Verification items for this drawing (mm, ordinates from the low corner). Coordinates: 2 decimals unless noted, no trailing zeros. Write each loop counter-clockwise with the first axis right and the second up, starting at its lowest first coordinate (ties: lowest second). Pieces come first, ordered by that corner, then holes. Notation, with made-up numbers: (62.5, -38) -> (92.5, -38) arc R17 cw to (92.5, -10) -> close; hole circle Ø11 at (58, 74.5). An arc over 180 degrees is marked (long way). One line per item, written item: value. Start each with the question number.
1) Sectioned sample at C-C on y = 1.75. Enter the section's corners in (x, z) (1 decimal).
2) Gauge pin test, flat ends, axial feed: P1, Ø6, axis at x = 156.31, z = 156.31, coming from the -Y side; P2, Ø3, axis at y = 8, z = 144.5, coming from the +X side (1 decimal); P3, Ø5, axis at y = 6, z = 56, coming from the +X side (1 decimal); P4, Ø3, axis at y = 6.5, z = 106.5, coming from the +X side (1 decimal). Record the tip position at first contact, or that the pin passes through.
3) Sectioned sample at B-B on z = 25. Enter the section's corners in (x, y) (1 decimal), plus the area to 3 significant figures.
4) Sectioned sample at D-D on x = 25. Enter the section's corners in (y, z) (1 decimal).
5) Scan lines: line 1 along X through (y, z) = (1.75, 139.5) (1 decimal); line 2 along X through (y, z) = (7, 145) (1 decimal); line 3 along Z through (x, y) = (33, 4.25) (1 decimal). Record each from-to range of solid material in increasing order. Write a range as [from, to].
6) Sectioned sample at A-A on x = 167.5. Enter the section's corners in (y, z) (1 decimal).
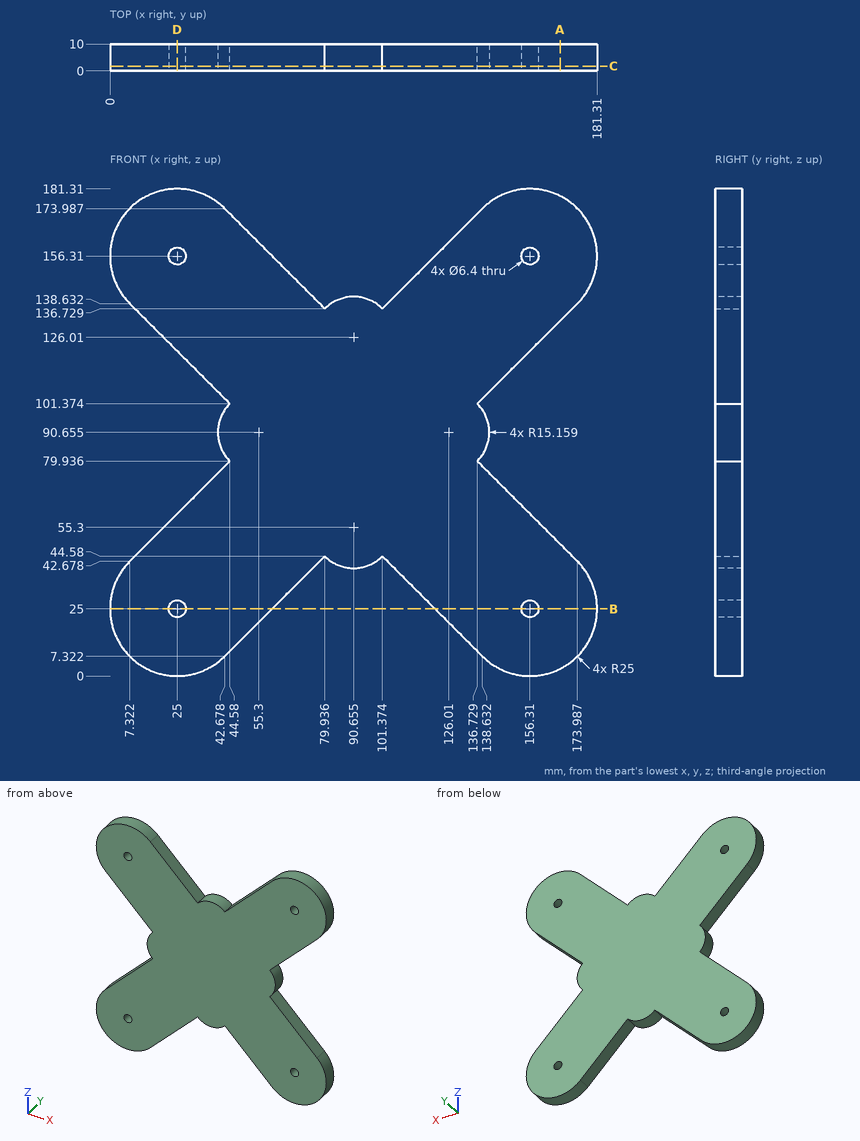
Answers:
1. outline: (7.3, 42.7) arc R25 ccw to (42.7, 7.3) -> (79.9, 44.6) arc R15.2 ccw to (101.4, 44.6) -> (138.6, 7.3) arc R25 ccw to (174, 42.7) -> (136.7, 79.9) arc R15.2 ccw to (136.7, 101.4) -> (174, 138.6) arc R25 ccw to (138.6, 174) -> (101.4, 136.7) arc R15.2 ccw to (79.9, 136.7) -> (42.7, 174) arc R25 ccw to (7.3, 138.6) -> (44.6, 101.4) arc R15.2 ccw to (44.6, 79.9) -> close; hole circle Ø6.4 at (25, 25); hole circle Ø6.4 at (25, 156.3); hole circle Ø6.4 at (156.3, 25); hole circle Ø6.4 at (156.3, 156.3)
2. P1: passes through
2. P2: stops at x = 179.1
2. P3: stops at x = 163.2
2. P4: stops at x = 143.4
3. outline: (0, 0) -> (21.8, 0) -> (21.8, 10) -> (0, 10) -> close; (28.2, 0) -> (60.4, 0) -> (60.4, 10) -> (28.2, 10) -> close; (121, 0) -> (153.1, 0) -> (153.1, 10) -> (121, 10) -> close; (159.5, 0) -> (181.3, 0) -> (181.3, 10) -> (159.5, 10) -> close
3. area: 1,080 mm2
4. outline: (0, 0) -> (10, 0) -> (10, 21.8) -> (0, 21.8) -> close; (0, 28.2) -> (10, 28.2) -> (10, 60.4) -> (0, 60.4) -> close; (0, 121) -> (10, 121) -> (10, 153.1) -> (0, 153.1) -> close; (0, 159.5) -> (10, 159.5) -> (10, 181.3) -> (0, 181.3) -> close
5. line 1: x = [6.5, 77.2], [83.7, 97.6], [104.1, 174.8]
5. line 2: x = [2.7, 71.7], [109.6, 178.6]
5. line 3: z = [1.3, 68.4], [113, 180]
6. outline: (0, 2.6) -> (10, 2.6) -> (10, 49.2) -> (0, 49.2) -> close; (0, 132.1) -> (10, 132.1) -> (10, 178.7) -> (0, 178.7) -> close
